Input: part model. Units: mm. Frame: model coordinates. A direction names the side the tool comes from. Coordinates: 2 decimals unless noted, no trailing zeros. Order: outer loops, then holes, each group sorted by start corner. A loop starts at its lowest first (then second) coordinate and runs counter-clockwise, first axis right, second up.
from build123d import *

# Parameters (mm, degrees)
IZIM1_W                     = 300
IZIM1_H                     = 300
Y_KSEKLIK_EKSTR_ZYON1_DEPTH = 200
BO_ALTMA1_T                 = -4
KES_EKSTR_ZYON1_REACH       = 471.042
IZIM2_R                     = 4
KES_EKSTR_ZYON2_REACH       = 471.042
IZIM3_R                     = 4
IZIM3_R_2                   = 2


with BuildPart() as part:
    # izim1 → Y_kseklik-Ekstr_zyon1 (new body)
    with BuildSketch(Plane.XY):
        with Locations((-150, 150)):
            Rectangle(IZIM1_W, IZIM1_H)
    extrude(amount=Y_KSEKLIK_EKSTR_ZYON1_DEPTH)

    # Bo_altma1
    bo_altma1_openings = [part.faces().sort_by_distance(p)[0] for p in [
        (-150, 150, 200),
    ]]
    offset(amount=BO_ALTMA1_T, openings=bo_altma1_openings, kind=Kind.INTERSECTION)

    # izim2 → Kes-Ekstr_zyon1 (cut, up to next)
    with BuildSketch(Plane.ZY.offset(300), mode=Mode.PRIVATE) as kes_ekstr_zyon1_sk1:
        with Locations((146.25, 250)):
            Circle(IZIM2_R)
    kes_ekstr_zyon1_tool1 = extrude(kes_ekstr_zyon1_sk1.sketch, amount=-KES_EKSTR_ZYON1_REACH, mode=Mode.PRIVATE) & part.part
    # izim2 → Kes-Ekstr_zyon1 (cut, up to next)
    with BuildSketch(Plane.ZY.offset(300), mode=Mode.PRIVATE) as kes_ekstr_zyon1_sk2:
        with Locations((53.75, 250)):
            Circle(IZIM2_R)
    kes_ekstr_zyon1_tool2 = extrude(kes_ekstr_zyon1_sk2.sketch, amount=-KES_EKSTR_ZYON1_REACH, mode=Mode.PRIVATE) & part.part
    # izim2 → Kes-Ekstr_zyon1 (cut, up to next)
    with BuildSketch(Plane.ZY.offset(300), mode=Mode.PRIVATE) as kes_ekstr_zyon1_sk3:
        with Locations((146.25, 157.5)):
            Circle(IZIM2_R)
    kes_ekstr_zyon1_tool3 = extrude(kes_ekstr_zyon1_sk3.sketch, amount=-KES_EKSTR_ZYON1_REACH, mode=Mode.PRIVATE) & part.part
    # izim2 → Kes-Ekstr_zyon1 (cut, up to next)
    with BuildSketch(Plane.ZY.offset(300), mode=Mode.PRIVATE) as kes_ekstr_zyon1_sk4:
        with Locations((53.75, 157.5)):
            Circle(IZIM2_R)
    kes_ekstr_zyon1_tool4 = extrude(kes_ekstr_zyon1_sk4.sketch, amount=-KES_EKSTR_ZYON1_REACH, mode=Mode.PRIVATE) & part.part
    kes_ekstr_zyon1_1 = kes_ekstr_zyon1_tool1.solids().sort_by_distance((-300, 250, 146.25))[0]
    add(kes_ekstr_zyon1_1, mode=Mode.SUBTRACT)
    kes_ekstr_zyon1_2 = kes_ekstr_zyon1_tool2.solids().sort_by_distance((-300, 250, 53.75))[0]
    add(kes_ekstr_zyon1_2, mode=Mode.SUBTRACT)
    kes_ekstr_zyon1_3 = kes_ekstr_zyon1_tool3.solids().sort_by_distance((-300, 157.5, 146.25))[0]
    add(kes_ekstr_zyon1_3, mode=Mode.SUBTRACT)
    kes_ekstr_zyon1_4 = kes_ekstr_zyon1_tool4.solids().sort_by_distance((-300, 157.5, 53.75))[0]
    add(kes_ekstr_zyon1_4, mode=Mode.SUBTRACT)
    kes_ekstr_zyon1 = kes_ekstr_zyon1_1 + kes_ekstr_zyon1_2 + kes_ekstr_zyon1_3 + kes_ekstr_zyon1_4  # Kes-Ekstr_zyon1 as one shape, for the pattern or mirror that repeats it

    # Aynalama1: Kes-Ekstr_zyon1 across plane
    add(kes_ekstr_zyon1.mirror(Plane(origin=(-150, 0, 0), x_dir=(0, 0, 1), z_dir=(1, 0, 0))), mode=Mode.SUBTRACT)

    # izim3 → Kes-Ekstr_zyon2 (cut, up to next)
    with BuildSketch(Plane.XZ, mode=Mode.PRIVATE) as kes_ekstr_zyon2_sk1:
        with Locations(Location((-150, 100, 0), (0, 0, 270))):
            Circle(IZIM3_R)
    kes_ekstr_zyon2_tool1 = extrude(kes_ekstr_zyon2_sk1.sketch, amount=-KES_EKSTR_ZYON2_REACH, mode=Mode.PRIVATE) & part.part
    # izim3 → Kes-Ekstr_zyon2 (cut, up to next)
    with BuildSketch(Plane.XZ, mode=Mode.PRIVATE) as kes_ekstr_zyon2_sk2:
        with Locations(Location((-150, 108, 0), (0, 0, 270))):
            Circle(IZIM3_R_2)
    kes_ekstr_zyon2_tool2 = extrude(kes_ekstr_zyon2_sk2.sketch, amount=-KES_EKSTR_ZYON2_REACH, mode=Mode.PRIVATE) & part.part
    # izim3 → Kes-Ekstr_zyon2 (cut, up to next)
    with BuildSketch(Plane.XZ, mode=Mode.PRIVATE) as kes_ekstr_zyon2_sk3:
        with Locations(Location((-158, 100, 0), (0, 0, 270))):
            Circle(IZIM3_R_2)
    kes_ekstr_zyon2_tool3 = extrude(kes_ekstr_zyon2_sk3.sketch, amount=-KES_EKSTR_ZYON2_REACH, mode=Mode.PRIVATE) & part.part
    # izim3 → Kes-Ekstr_zyon2 (cut, up to next)
    with BuildSketch(Plane.XZ, mode=Mode.PRIVATE) as kes_ekstr_zyon2_sk4:
        with Locations(Location((-150, 92, 0), (0, 0, 270))):
            Circle(IZIM3_R_2)
    kes_ekstr_zyon2_tool4 = extrude(kes_ekstr_zyon2_sk4.sketch, amount=-KES_EKSTR_ZYON2_REACH, mode=Mode.PRIVATE) & part.part
    # izim3 → Kes-Ekstr_zyon2 (cut, up to next)
    with BuildSketch(Plane.XZ, mode=Mode.PRIVATE) as kes_ekstr_zyon2_sk5:
        with Locations(Location((-142, 100, 0), (0, 0, 270))):
            Circle(IZIM3_R_2)
    kes_ekstr_zyon2_tool5 = extrude(kes_ekstr_zyon2_sk5.sketch, amount=-KES_EKSTR_ZYON2_REACH, mode=Mode.PRIVATE) & part.part
    add(kes_ekstr_zyon2_tool1.solids().sort_by_distance((-150, 0, 100))[0], mode=Mode.SUBTRACT)
    add(kes_ekstr_zyon2_tool2.solids().sort_by_distance((-150, 0, 108))[0], mode=Mode.SUBTRACT)
    add(kes_ekstr_zyon2_tool3.solids().sort_by_distance((-158, 0, 100))[0], mode=Mode.SUBTRACT)
    add(kes_ekstr_zyon2_tool4.solids().sort_by_distance((-150, 0, 92))[0], mode=Mode.SUBTRACT)
    add(kes_ekstr_zyon2_tool5.solids().sort_by_distance((-142, 0, 100))[0], mode=Mode.SUBTRACT)


solid = part.part
Item 1: Draft query along Z for faces 4 (the face through (-152, 152, 0)), 5 (the face through (-1.972, 253.373, 55.9)), 6 (the face through (-296, 148, 101)), 7 (the face through (-152, 152, 4)). Return one class per face: pulls with the +Z half, pulls with the -Z half, needs draft (parallel to the pull), parting line crosses it, or undercut.
Response values:
face 4: pulls with the -Z half
face 5: undercut
face 6: needs draft
face 7: pulls with the +Z half
Item 2: Cut plane A-A on z = 53.75. Return loops of the section in (x, y).
Response values:
outline: (-300, 0) - (0, 0) - (0, 153.5) - (-4, 153.5) - (-4, 4) - (-296, 4) - (-296, 153.5) - (-300, 153.5) - close; (-300, 161.5) - (-296, 161.5) - (-296, 246) - (-300, 246) - close; (-300, 254) - (-296, 254) - (-296, 296) - (-4, 296) - (-4, 254) - (0, 254) - (0, 300) - (-300, 300) - close; (-4, 161.5) - (0, 161.5) - (0, 246) - (-4, 246) - close
Item 3: Cut plane C-C on z = 14.5. Return loops of the section in (x, y), then the cut area to 3 significant figures.
Response values:
outline: (-300, 0) - (0, 0) - (0, 300) - (-300, 300) - close; hole (-296, 4) - (-4, 4) - (-4, 296) - (-296, 296) - close
area: 4,740 mm2
Item 4: Cut plane B-B on y = 250. Return loops of the section in (x, z).
Response values:
outline: (-300, 0) - (0, 0) - (0, 49.75) - (-4, 49.75) - (-4, 4) - (-296, 4) - (-296, 49.75) - (-300, 49.75) - close; (-300, 57.75) - (-296, 57.75) - (-296, 142.25) - (-300, 142.25) - close; (-300, 150.25) - (-296, 150.25) - (-296, 200) - (-300, 200) - close; (-4, 57.75) - (0, 57.75) - (0, 142.25) - (-4, 142.25) - close; (-4, 150.25) - (0, 150.25) - (0, 200) - (-4, 200) - close
Item 5: Cut plane D-D on x = -190. Return loops of the section in (y, z), then the cut area to 3 significant figures.
Response values:
outline: (0, 0) - (300, 0) - (300, 200) - (296, 200) - (296, 4) - (4, 4) - (4, 200) - (0, 200) - close
area: 2,770 mm2
Item 6: Pin query (flat end, axial travel): pin 1 Ø5 at (x, z) = (-141.5, 147) entering from -Y; pin 2 Ø12 at (x, y) = (-211.5, 80.5) entering from +Z. Return the tip coordinate at first contact, or that it passes through.
Response values:
pin 1: stops at y = 0
pin 2: stops at z = 4
Item 7: Access query for faces 1 (the face through (-146.034, 1.972, 100.521)), 2 (the face through (-152, 296, 101)), 3 (the face through (-1.972, 160.873, 148.4)). Directions: +Z, -Z, +X, -X, +Y, -Y. A direction counts if a zero-diameter tool reaches every point of the face in a straight line with its end or side. Return the directions, or none.
Response values:
face 1: -Y
face 2: +Z
face 3: +X, -X
Item 8: Ray query, probe 1 along Y at (x, z) = (-1, 146); probe 2 along Z at (x, y) = (-1, 157); probe 3 along X at (y, z) = (231, 133). Return the intervals inside material, ascending.
Response values:
probe 1: y = 0 to 153.51, 161.49 to 246.01, 253.99 to 300
probe 2: z = 0 to 49.78, 57.72 to 142.28, 150.22 to 200
probe 3: x = -300 to -296, -4 to 0
